```python
from build123d import *

# Parameters (mm, degrees)
SKETCH1_R               = 12.7
BOSS_EXTRUDE1_DEPTH     = 9
SKETCH2_R               = 17.7
BOSS_EXTRUDE2_DEPTH     = 3
SKETCH3_R               = 3.1
SKETCH3_R_2             = 1.58
CUT_EXTRUDE1_DEPTH      = 10
CUT_EXTRUDE1_DEPTH_BACK = 4
SKETCH4_R               = 3.1
BOSS_EXTRUDE3_DEPTH     = 5.5
SKETCH5_W               = 6.2
SKETCH5_H               = 1.8
BOSS_EXTRUDE4_DEPTH     = 6.5


with BuildPart() as part:
    # Sketch1 → Boss-Extrude1 (new body)
    with BuildSketch(Plane(origin=(0, 0, 0), x_dir=(1, 0, 0), z_dir=(0, 1, 0))):
        Circle(SKETCH1_R)
    extrude(amount=BOSS_EXTRUDE1_DEPTH)

    # Sketch2 → Boss-Extrude2 (add)
    with BuildSketch(Plane(origin=(0, 0, 0), x_dir=(-1, 0, 0), z_dir=(0, 1, 0))):
        Circle(SKETCH2_R)
    extrude(amount=-BOSS_EXTRUDE2_DEPTH)

    # Sketch3 → Cut-Extrude1 (cut, two sides)
    with BuildSketch(Plane(origin=(0, 0, 0), x_dir=(1, 0, 0), z_dir=(0, 1, 0))) as cut_extrude1_sk:
        Circle(SKETCH3_R)
        with Locations((-9, 0)):
            Circle(SKETCH3_R_2)
        with Locations((9, 0)):
            Circle(SKETCH3_R_2)
        with Locations((0, 9)):
            Circle(SKETCH3_R_2)
        with Locations((0, -9)):
            Circle(SKETCH3_R_2)
    extrude(amount=CUT_EXTRUDE1_DEPTH, mode=Mode.SUBTRACT)
    extrude(cut_extrude1_sk.sketch, amount=-CUT_EXTRUDE1_DEPTH_BACK, mode=Mode.SUBTRACT)

    # Sketch4 → Boss-Extrude3 (add)
    with BuildSketch(Plane.XZ.offset(3)):
        Circle(SKETCH4_R)
    extrude(amount=-BOSS_EXTRUDE3_DEPTH)

    # Sketch5 → Boss-Extrude4 (add)
    with BuildSketch(Plane(origin=(0, 9, 0), x_dir=(1, 0, 0), z_dir=(0, 1, 0))):
        with Locations((0, 2.2)):
            Rectangle(SKETCH5_W, SKETCH5_H)
    extrude(amount=-BOSS_EXTRUDE4_DEPTH)


solid = part.part
```
Design review of the part built by this model. Coordinates are the model's own, in mm. A direction names the side the tool comes from. Coordinates: 2 decimals unless noted, no trailing zeros. Order: outer loops, then holes, each group sorted by start corner. A loop starts at its lowest first (then second) coordinate and runs counter-clockwise, first axis right, second up. Notation, with made-up numbers: M 73.25,61 L 112.25,61 A11 cw 112.25,81 Z; hole C 42,29 d6. An arc over 180 degrees is marked long. Answer as a JSON object with one key per item and string values. Group by question number.
1) For pin 1 (3.5 mm diameter, centred on x = 9, z = 0, fed in from -Y); pin 2 (3 mm diameter, centred on x = -1, y = 7, fed in from +Z); pin 3 (1 mm diameter, centred on x = 4, y = -1.5, fed in from +Z), all flat-tipped, find the tip position at first contact; note any pin that passes through.
2) Add section C-C, the plane y = 4. Write out the cut boundary in (x, z).
3) Add section A-A, the plane x = 0. Write out the cut boundary in (y, z), then the cut area to 3 significant figures.
4) Add section B-B, the plane z = 9. Write out the cut boundary in (x, y), then the cut area to 3 significant figures.
5) Add section D-D, the plane y = 0.5. Write out the cut boundary in (x, z).
6) Wall thickness on L1, parallel to X at y = 4, z = 0; L2, parallel to Z at x = 0, y = 1; L3, parallel to X at y = 3.5, z = -1: over which ranges is each line inside the solid? List them lowest first.
7) Tool access review of faces 1 (the cylindrical face through (-0.206, 3.084, 7.433)), 2 (the flat face through (0, 2.5, 0)): name each direction out of +Z, -Z, +X, -X, +Y, -Y from which nothing blocks a thin tool from reaching the whole face with its end or side.
8) Mouldability with a two-part tool opening along Z and no side actions: class faces 3 (the flat face through (0, -3, 0)), 4 (the flat face through (0, 6, -1.3)), 5 (the cylindrical face through (-16.88, -1.48, 5.32)) as pulls with the +Z half, pulls with the -Z half, needs draft (parallel to the pull), parting line crosses it, or undercut.
Computed values:
{
 "1": {"pin 1": "stops at y = -3", "pin 2": "stops at z = 12.7", "pin 3": "stops at z = 17.35"},
 "2": {"outline": "C 0,0 d25.4; hole C -9,0 d3.16; hole M -2.81,-1.3 L 2.81,-1.3 A3.1 ccw long Z; hole C 0,-9 d3.16; hole C 0,9 d3.16; hole C 9,0 d3.16"},
 "3": {"outline": "M -3,-17.7 L 0,-17.7 L 0,-12.7 L 9,-12.7 L 9,-10.58 L -3,-10.58 Z; M -3,-7.42 L 9,-7.42 L 9,-1.3 L 2.5,-1.3 L 2.5,3.1 L 9,3.1 L 9,7.42 L -3,7.42 Z; M -3,10.58 L 9,10.58 L 9,12.7 L 0,12.7 L 0,17.7 L -3,17.7 Z", "area": "230 mm^2"},
 "4": {"outline": "M -15.24,-3 L -1.58,-3 L -1.58,9 L -8.96,9 L -8.96,0 L -15.24,0 Z; M 1.58,-3 L 15.24,-3 L 15.24,0 L 8.96,0 L 8.96,9 L 1.58,9 Z", "area": "215 mm^2"},
 "5": {"outline": "C 0,0 d25.4; hole C -9,0 d3.16; hole C 0,-9 d3.16; hole C 0,9 d3.16; hole C 9,0 d3.16"},
 "6": {"L1": "x = -12.7 to -10.58, -7.42 to -3.1, 3.1 to 7.42, 10.58 to 12.7", "L2": "z = -12.7 to -10.58, -7.42 to 7.42, 10.58 to 12.7", "L3": "x = -12.66 to -10.22, -7.78 to -2.93, 2.93 to 7.78, 10.22 to 12.66"},
 "7": {"face 1": "+Y, -Y", "face 2": "+Y"},
 "8": {"face 3": "needs draft", "face 4": "undercut", "face 5": "parting line crosses it"}
}
